```python
from build123d import *

# Parameters (mm, degrees)
SKETCH1_W                = 50
SKETCH1_H                = 8
SKETCH1_R                = 1.5
BOSS_EXTRUDE1_DEPTH      = 4
SKETCH2_W                = 50
SKETCH2_H                = 2
BOSS_EXTRUDE2_DEPTH      = 30
BOSS_EXTRUDE2_DEPTH_BACK = 4
SKETCH3_W                = 2
SKETCH3_H                = 30
BOSS_EXTRUDE3_DEPTH      = 50
FILLET1_R                = 10
FILLET2_R                = 5
FILLET3_R                = 1.5
SKETCH4_R                = 1.625
CUT_EXTRUDE1_DEPTH       = 13


with BuildPart() as part:
    # Sketch1 → Boss-Extrude1 (new body)
    with BuildSketch(Plane.XY):
        with Locations((-29.042911783, 15.053723554)):
            Rectangle(SKETCH1_W, SKETCH1_H)
        with Locations((-41.180553897, 15.053723554)):
            Circle(SKETCH1_R, mode=Mode.SUBTRACT)
        with Locations((-16.905269669, 15.053723554)):
            Circle(SKETCH1_R, mode=Mode.SUBTRACT)
    extrude(amount=BOSS_EXTRUDE1_DEPTH)

    # Sketch2 → Boss-Extrude2 (add, two sides)
    with BuildSketch(Plane.XY.offset(4)) as boss_extrude2_sk:
        with Locations((-29.042911783, 20.053723554)):
            Rectangle(SKETCH2_W, SKETCH2_H)
    extrude(amount=BOSS_EXTRUDE2_DEPTH)
    extrude(boss_extrude2_sk.sketch, amount=-BOSS_EXTRUDE2_DEPTH_BACK)

    # Sketch3 → Boss-Extrude3 (add)
    with BuildSketch(Plane.ZY.offset(54.042911783)):
        with Locations((35, 34.053723554)):
            Rectangle(SKETCH3_W, SKETCH3_H)
    extrude(amount=-BOSS_EXTRUDE3_DEPTH)

    # Fillet1
    fillet1_edges = [part.edges().sort_by_distance(p)[0] for p in [
        (-4.042911783, 49.053723554, 35),
        (-54.042911783, 49.053723554, 35),
    ]]
    fillet(fillet1_edges, radius=FILLET1_R)

    # Fillet2
    fillet2_edges = [part.edges().sort_by_distance(p)[0] for p in [
        (-54.042911783, 11.053723554, 2),
        (-4.042911783, 11.053723554, 2),
    ]]
    fillet(fillet2_edges, radius=FILLET2_R)

    # Fillet3
    fillet3_edges = [part.edges().sort_by_distance(p)[0] for p in [
        (-29.042911783, 21.053723554, 34),
        (-29.042911783, 19.053723554, 36),
    ]]
    fillet(fillet3_edges, radius=FILLET3_R)

    # Sketch4 → Cut-Extrude1 (cut)
    with BuildSketch(Plane.XY.offset(36)):
        with Locations((-24.367911783, 46.053723554)):
            Circle(SKETCH4_R)
        with Locations((-33.717911783, 46.053723554)):
            Circle(SKETCH4_R)
    extrude(amount=-CUT_EXTRUDE1_DEPTH, mode=Mode.SUBTRACT)


solid = part.part
```
Work out the finished part from the listing and answer in its coordinate system (mm). A direction names the side the tool comes from. Coordinates: 2 decimals unless noted, no trailing zeros. Loops run counter-clockwise (first coordinate to the right, second up) from the corner with the lowest first, then second, coordinate; pieces in that order, holes last.
1) For a pull along X with two mould halves and no side action, classify faces 1 (the cylindrical face through (-42.68, 15.12, 1.97)), 2 (the flat face through (-4.043, 20.8, 19.2)), 3 (the cylindrical face through (-28.69, 19.48, 35.55)) as +X half, -X half, draft (parallel to the pull), parting line (faces both ways), or undercut.
Results:
face 1: undercut
face 2: +X half
face 3: draft
2) For faces 4 (the flat face through (-29, 11.054, 2)), 5 (the flat face through (-29, 21.054, 16)), 6 (the flat face through (-29, 19.054, 19)), determine the directions among +Z, -Z, +X, -X, +Y, -Y from which every point of the face is accessible in a straight line to the end or side of a thin tool.
Results:
face 4: +Z, -Z, +X, -X, -Y
face 5: -Z, +X, -X, +Y
face 6: +Z, +X, -X, -Y
3) Section B-B (x = -37) is taken. Give the vertices of the cut face in (y, z), plus the area to 3 significant figures.
Results:
outline: (11.05, 0) - (21.05, 0) - (21.05, 32.5) arc R1.5 cw to (22.55, 34) - (49.05, 34) - (49.05, 36) - (20.55, 36) arc R1.5 ccw to (19.05, 34.5) - (19.05, 4) - (11.05, 4) - close
area: 160 mm2
4) Section D-D (z = 31) is taken. Give the vertices of the cut face in (x, y), plus the area to 3 significant figures.
Results:
outline: (-54.04, 19.05) - (-4.04, 19.05) - (-4.04, 21.05) - (-54.04, 21.05) - close
area: 100 mm2
5) Consider probe 1 along Y at (x, z) = (-44, 14); probe 2 along Z at (x, y) = (-40.5, 37.5); probe 3 along Z at (x, y) = (-32, 17). Determine where each line is inside the solid, lowest interval first.
Results:
probe 1: y = 19.05 to 21.05
probe 2: z = 34 to 36
probe 3: z = 0 to 4
6) Flat-ended cylindrical pins translate along their axes: pin 1 (10 mm diameter, centred on x = -33, z = 17.5, fed in from +Y); pin 2 (4 mm diameter, centred on x = -16.91, y = 15.05, fed in from -Z); pin 3 (5 mm diameter, centred on x = -24.37, y = 46.05, fed in from -Z); pin 4 (5 mm diameter, centred on x = -41.18, y = 15.05, fed in from +Z). Find the tip coordinate at first contact, or state that the pin passes through.
Results:
pin 1: stops at y = 21.05
pin 2: stops at z = 0
pin 3: stops at z = 34
pin 4: stops at z = 4
7) Section C-C (y = 29.5) is taken. Give the vertices of the cut face in (x, z).
Results:
outline: (-54.04, 34) - (-4.04, 34) - (-4.04, 36) - (-54.04, 36) - close
8) Section A-A (x = -24) is taken. Give the vertices of the cut face in (y, z), plus the area to 3 significant figures.
Results:
outline: (11.05, 0) - (21.05, 0) - (21.05, 32.5) arc R1.5 cw to (22.55, 34) - (44.47, 34) - (44.47, 36) - (20.55, 36) arc R1.5 ccw to (19.05, 34.5) - (19.05, 4) - (11.05, 4) - close; (47.64, 34) - (49.05, 34) - (49.05, 36) - (47.64, 36) - close
area: 154 mm2
